```python
from build123d import *

# Parameters (mm, degrees)
SKETCH005_R      = 6
EXTRUDE005_DEPTH = 1.75
SKETCH004_R      = 1.25
EXTRUDE004_DEPTH = 1.75
SKETCH003_R      = 2
SKETCH003_R_2    = 15
EXTRUDE003_DEPTH = 1.75
SKETCH002_R      = 1.499044
EXTRUDE002_DEPTH = 1.75
SKETCH001_R      = 101.870707
EXTRUDE001_DEPTH = 1.75
EXTRUDE_DEPTH    = 1.75
FILLET001_R      = 2.5


with BuildPart() as obj1:
    # Sketch005 (on Cut) → Extrude005 (new body)
    with BuildSketch(Plane.XY.offset(-1.75)):
        with Locations((-33, -33)):
            Circle(SKETCH005_R)
        with Locations((33, -33)):
            Circle(SKETCH005_R)
        with Locations((33, 33)):
            Circle(SKETCH005_R)
        with Locations((-33, 33)):
            Circle(SKETCH005_R)
    extrude(amount=EXTRUDE005_DEPTH)


with BuildPart() as obj1_1:
    # Extrude005 placement: moved
    add(obj1.part.moved(Location((0, 0, 39.25))))


with BuildPart() as obj2:
    # Sketch004 (on Face2 of Cut002) → Extrude004 (new body)
    with BuildSketch(Plane(origin=(0, 0, 39.25), x_dir=(1, 0, 0), z_dir=(0, 0, -1))):
        with Locations((-18, -45)):
            Circle(SKETCH004_R)
        with Locations((18, -45)):
            Circle(SKETCH004_R)
        with Locations((18, 45)):
            Circle(SKETCH004_R)
        with Locations((-18, 45)):
            Circle(SKETCH004_R)
        with Locations((45, -18)):
            Circle(SKETCH004_R)
        with Locations((45, 18)):
            Circle(SKETCH004_R)
        with Locations((-45, -18)):
            Circle(SKETCH004_R)
        with Locations((-45, 18)):
            Circle(SKETCH004_R)
    extrude(amount=-EXTRUDE004_DEPTH)


with BuildPart() as pcb_mount_holes:
    # Sketch003 (on Face4 of Cut001) → Extrude003 (new body)
    with BuildSketch(Plane.XY.offset(41)):
        with Locations((0, -30)):
            Circle(SKETCH003_R)
        with Locations((-30, 0)):
            Circle(SKETCH003_R)
        with Locations((0, 30)):
            Circle(SKETCH003_R)
        with Locations((30, 0)):
            Circle(SKETCH003_R)
        Circle(SKETCH003_R_2)
    extrude(amount=EXTRUDE003_DEPTH)


with BuildPart() as pcb_mount_holes_1:
    # Extrude003 placement: moved
    add(pcb_mount_holes.part.moved(Location((0, 0, -1.75))))


with BuildPart() as new_plate_mount_holes:
    # Sketch002 (on Face4 of Cut) → Extrude002 (new body)
    with BuildSketch(Plane.XY.offset(41)):
        with Locations((-47.205132, 30.588341)):
            Circle(SKETCH002_R)
        with Locations((-30.567202, 47.199055)):
            Circle(SKETCH002_R)
        with Locations((-30.397604, 19.093531)):
            Circle(SKETCH002_R)
        with Locations((-19.088974, 30.411751)):
            Circle(SKETCH002_R)
        with Locations((19.10001, 30.403801)):
            Circle(SKETCH002_R)
        with Locations((30.583944, 47.210339)):
            Circle(SKETCH002_R)
        with Locations((30.394878, 19.093672)):
            Circle(SKETCH002_R)
        with Locations((47.19109, 30.57703)):
            Circle(SKETCH002_R)
        with Locations((30.412411, -19.089888)):
            Circle(SKETCH002_R)
        with Locations((47.194775, -30.584883)):
            Circle(SKETCH002_R)
        with Locations((19.091776, -30.4009)):
            Circle(SKETCH002_R)
        with Locations((30.581888, -47.195107)):
            Circle(SKETCH002_R)
        with Locations((-30.587105, -47.201801)):
            Circle(SKETCH002_R)
        with Locations((-19.094023, -30.403849)):
            Circle(SKETCH002_R)
        with Locations((-30.409216, -19.085772)):
            Circle(SKETCH002_R)
        with Locations((-47.198414, -30.583656)):
            Circle(SKETCH002_R)
    extrude(amount=EXTRUDE002_DEPTH)


with BuildPart() as new_plate_mount_holes_1:
    # Extrude002 placement: moved
    add(new_plate_mount_holes.part.moved(Location((0, 0, -1.75))))


with BuildPart() as new_plate_base_neg1:
    # Sketch001 (on Face9 of Extrude) → Extrude001 (new body)
    with BuildSketch(Plane(origin=(0, 0, 39.25), x_dir=(1, 0, 0), z_dir=(0, 0, -1))):
        with Locations((-0.000254, 150.000229)):
            Circle(SKETCH001_R)
        with Locations((150.009079, 0.007901)):
            Circle(SKETCH001_R)
        with Locations((-0.021678, -150.013428)):
            Circle(SKETCH001_R)
        with Locations((-150.015869, -0.046967)):
            Circle(SKETCH001_R)
    extrude(amount=-EXTRUDE001_DEPTH)


with BuildPart() as top_plate_new:
    # Sketch (on Face200 of F450107) → Extrude (new body)
    with BuildSketch(Plane.XY.offset(39.25)):
        Polygon((61.25, -25.370581), (61.25, 25.370581), (25.370581, 61.25), (-25.370581, 61.25), (-61.25, 25.370581), (-61.25, -25.370581), (-25.370581, -61.25), (25.370581, -61.25), align=None)
    extrude(amount=EXTRUDE_DEPTH)

    # Cut: cut new_plate_base_neg1
    add(new_plate_base_neg1.part, mode=Mode.SUBTRACT)

    # Cut001: cut new_plate_mount_holes
    add(new_plate_mount_holes_1.part, mode=Mode.SUBTRACT)

    # Cut002: cut pcb_mount_holes
    add(pcb_mount_holes_1.part, mode=Mode.SUBTRACT)

    # Cut003: cut obj2
    add(obj2.part, mode=Mode.SUBTRACT)


with BuildPart() as top_plate_new_1:
    # Cut003 placement: moved
    add(top_plate_new.part.moved(Location((0, 0, -1.75))))

    # Cut004: cut obj1
    add(obj1_1.part, mode=Mode.SUBTRACT)

    # Fillet001
    fillet001_edges = [top_plate_new_1.edges().sort_by_distance(p)[0] for p in [
        (53.626688, -32.993893, 38.375),
        (32.998406, -53.622175, 38.375),
        (53.630718, 32.989863, 38.375),
        (-32.998536, -53.622045, 38.375),
        (-53.645742, -32.974838, 38.375),
        (32.983109, 53.637472, 38.375),
        (-32.994165, 53.626416, 38.375),
        (-53.621791, 32.99879, 38.375),
    ]]
    fillet(fillet001_edges, radius=FILLET001_R)


solid = top_plate_new_1.part
```
Check sheet for the modelled part. Datum: model origin and axes. Units: mm. Give positions to 0.01 mm unless a question says otherwise; leave off trailing zeros. Write each loop counter-clockwise with the first axis right and the second up, starting at its lowest first coordinate (ties: lowest second). Pieces come first, ordered by that corner, then holes.
Item 1: Draft check along X on faces 1 (the face through (-19.414, 28.948, 38.363)), 2 (the face through (48.14, -0.45, 38.36)), 3 (the face through (-13, 13, 39.25)). Enter one of: released by +X, released by -X, zero draft, split by the parting line, or undercut.
Item 2: Cross-section at A-A (x = 0). Enter the section's corners in (y, z), and give its area (3 significant figures).
Item 3: Gauge pin test, flat ends, axial feed: pin 1 (1 mm diameter, centred on y = -16.5, z = 38, fed in from -X); pin 2 (11 mm diameter, centred on x = -33, y = 33, fed in from +Z). Record the tip position at first contact, or that the pin passes through.
Item 4: Cross-section at B-B (y = 5). Enter the section's corners in (x, z).
Item 5: Cross-section at C-C (z = 38.5). Count the separate pieces of the cut face and the enclosed holes in it, and give its area (3 significant figures).
Item 6: Scan lines: L1, parallel to X at y = 34.5, z = 39; L2, parallel to Y at x = 0, z = 37.8; L3, parallel to Y at x = -45, z = 38.2. Record each from-to range of solid material in increasing order.
Item 7: Cross-section at D-D (x = -25.5). Enter the section's corners in (y, z).
Report:
1. face 1: undercut
1. face 2: released by +X
1. face 3: zero draft
2. outline: (-48.13, 37.5) - (-32, 37.5) - (-32, 39.25) - (-48.13, 39.25) - close; (-28, 37.5) - (-15, 37.5) - (-15, 39.25) - (-28, 39.25) - close; (15, 37.5) - (28, 37.5) - (28, 39.25) - (15, 39.25) - close; (32, 37.5) - (48.14, 37.5) - (48.14, 39.25) - (32, 39.25) - close
2. area: 102 mm2
3. pin 1: stops at x = -49.58
3. pin 2: passes through
4. outline: (-48.27, 37.5) - (-14.14, 37.5) - (-14.14, 39.25) - (-48.27, 39.25) - close; (14.14, 37.5) - (48.26, 37.5) - (48.26, 39.25) - (14.14, 39.25) - close
5. separate pieces: 1
5. enclosed holes: 33
5. area: 8,320 mm2
6. L1: x = -52.12 to -38.81, -27.19 to 27.19, 38.81 to 52.12
6. L2: y = -48.13 to -32, -28 to -15, 15 to 28, 32 to 48.14
6. L3: y = -41.62 to -19.25, -16.75 to 16.75, 19.25 to 41.62
7. outline: (-51.37, 37.5) - (51.38, 37.5) - (51.38, 39.25) - (-51.37, 39.25) - close
